Read the model definition and answer for the solid it produces. Units are mm, in the model's axes. Coordinates: 2 decimals unless noted, no trailing zeros. Loops run counter-clockwise (first coordinate to the right, second up) from the corner with the lowest first, then second, coordinate; pieces in that order, holes last.
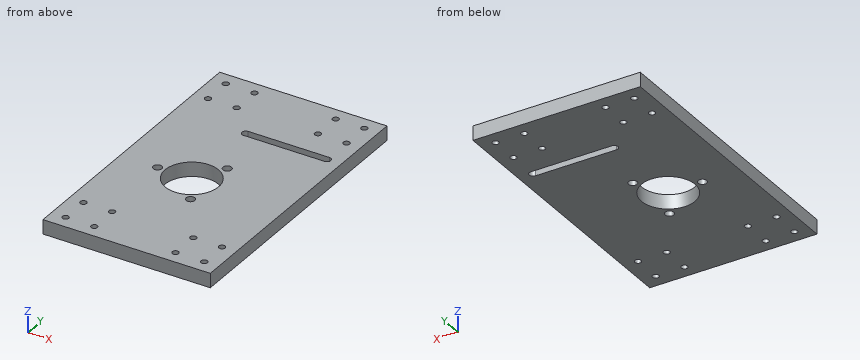
Solid Edge part; units mm, degrees
sketch "Sketch1" plane through (0, 0, 0) normal (0, 0, 1) x (1, 0, 0)
  line L0 (-123.7474, 0) -> (-123.7474, 300)
  line L1 (-123.7474, 300) -> (51.2526, 300)
  line L2 (51.2526, 300) -> (51.2526, 0)
  line L3 (51.2526, 0) -> (-123.7474, 0)
extrude "Protrusion1" add sketch "Sketch1" along normal blind 15
sketch "Sketch2" plane through (-248.7474, 300, 15) normal (0, 0, 1) x (1, 0, 0)
  circle A0 centre (200, -169) radius 28
  dimension "D1" = 200
extrude "Cutout1" cut sketch "Sketch2" against normal through all
hole "Hole_17" at (-30.8724, 100.0396, 15) direction (0, 0, -1) diameter 9 end up to next
hole "Hole1" at (-84.4974, 131, 15) direction (0, 0, -1) diameter 9 end up to next
hole "Hole2" at (-30.8724, 161.9604, 15) direction (0, 0, -1) diameter 9 end up to next
hole "Hole_9" at (36.2526, 45, 15) direction (0, 0, -1) diameter 6.6 end up to next
hole "Hole3" at (-108.7474, 45, 15) direction (0, 0, -1) diameter 6.6 end up to next
hole "Hole4" at (-108.7474, 15, 15) direction (0, 0, -1) diameter 6.6 end up to next
hole "Hole5" at (-108.7474, 255, 15) direction (0, 0, -1) diameter 6.6 end up to next
hole "Hole6" at (-108.7474, 285, 15) direction (0, 0, -1) diameter 6.6 end up to next
hole "Hole7" at (36.2526, 285, 15) direction (0, 0, -1) diameter 6.6 end up to next
hole "Hole8" at (36.2526, 255, 15) direction (0, 0, -1) diameter 6.6 end up to next
hole "Hole9" at (36.2526, 15, 15) direction (0, 0, -1) diameter 6.6 end up to next
hole "Hole10" at (6.2526, 15, 15) direction (0, 0, -1) diameter 6.6 end up to next
hole "Hole11" at (6.2526, 45, 15) direction (0, 0, -1) diameter 6.6 end up to next
hole "Hole12" at (-78.7474, 15, 15) direction (0, 0, -1) diameter 6.6 end up to next
hole "Hole13" at (-78.7474, 45, 15) direction (0, 0, -1) diameter 6.6 end up to next
hole "Hole14" at (6.2526, 255, 15) direction (0, 0, -1) diameter 6.6 end up to next
hole "Hole15" at (6.2526, 285, 15) direction (0, 0, -1) diameter 6.6 end up to next
hole "Hole16" at (-78.7474, 255, 15) direction (0, 0, -1) diameter 6.6 end up to next
hole "Hole17" at (-78.7474, 285, 15) direction (0, 0, -1) diameter 6.6 end up to next
sketch "Sketch3" plane through (-23.7474, 150, 15) normal (0, 0, 1) x (-1, 0, 0)
  circle A0 centre (-60, -72) radius 4
  circle A1 centre (25, -72) radius 4
  line L0 (-60, -68) -> (-60, -76)
  line L1 (-60, -76) -> (25, -76)
  line L2 (25, -76) -> (25, -68)
  line L3 (25, -68) -> (-60, -68)
  dimension "D1" = 25
extrude "Cutout2" cut sketch "Sketch3" against normal through all
sketch "Sketch4" plane through (-36.2474, 150, 0) normal (0, 0, -1) x (1, 0, 0)
  line L0 (-110.52, -149) -> (154.44, -149)
  line L1 (154.44, -149) -> (154.44, -163.44)
  line L2 (154.44, -163.44) -> (-110.52, -163.44)
  line L3 (-110.52, -163.44) -> (-110.52, -149)
  line L4 (-104.04, 177.84) -> (-104.04, 149)
  line L5 (-104.04, 149) -> (129.24, 149)
  line L6 (129.24, 149) -> (129.24, 177.84)
  line L7 (129.24, 177.84) -> (-104.04, 177.84)
extrude "Cutout3" cut sketch "Sketch4" against normal through all
properties material "Aluminum, 6061-T6"
Item 1: A cutting plane is placed at C-C on x = -58. Determine the outline of the cut face in (y, z), then the cut area to 3 significant figures.
Numbers:
outline: (1, 0) - (104.57, 0) - (104.57, 15) - (1, 15) - close; (157.43, 0) - (299, 0) - (299, 15) - (157.43, 15) - close
area: 3,680 mm2
Item 2: A cutting plane is placed at A-A on y = 15. Determine the outline of the cut face in (x, z), then the cut area to 3 significant figures.
Numbers:
outline: (-123.75, 0) - (-112.05, 0) - (-112.05, 15) - (-123.75, 15) - close; (-105.45, 0) - (-82.05, 0) - (-82.05, 15) - (-105.45, 15) - close; (-75.45, 0) - (2.95, 0) - (2.95, 15) - (-75.45, 15) - close; (9.55, 0) - (32.95, 0) - (32.95, 15) - (9.55, 15) - close; (39.55, 0) - (51.25, 0) - (51.25, 15) - (39.55, 15) - close
area: 2,230 mm2
Item 3: A cutting plane is placed at B-B on y = 131. Determine the outline of the cut face in (x, z).
Numbers:
outline: (-123.75, 0) - (-89, 0) - (-89, 15) - (-123.75, 15) - close; (-80, 0) - (-76.75, 0) - (-76.75, 15) - (-80, 15) - close; (-20.75, 0) - (51.25, 0) - (51.25, 15) - (-20.75, 15) - close
Item 4: Find the intervals of material crossed by line 1 along X through (y, z) = (255, 8.5); line 2 along Y through (x, z) = (-78.5, 14); line 3 along Y through (x, z) = (9, 2.25), in increasing order.
Numbers:
line 1: x = -123.75 to -112.05, -105.45 to -82.05, -75.45 to 2.95, 9.55 to 32.95, 39.55 to 51.25
line 2: y = 1 to 11.71, 18.29 to 41.71, 48.29 to 251.71, 258.29 to 281.71, 288.29 to 299
line 3: y = 1 to 13.17, 16.83 to 43.17, 46.83 to 218, 226 to 253.17, 256.83 to 283.17, 286.83 to 299
Item 5: Given pin 1 (4 mm diameter, centred on x = 6.25, y = 285, fed in from -Z), flat-ended and moving along its own axis, determine where the tip first touches the part or whether it passes through.
Numbers:
pin 1: passes through
Item 6: A cutting plane is placed at D-D on y = 222. Determine the outline of the cut face in (x, z).
Numbers:
outline: (-123.75, 0) - (-52.75, 0) - (-52.75, 15) - (-123.75, 15) - close; (40.25, 0) - (51.25, 0) - (51.25, 15) - (40.25, 15) - close
